CAD build for the part. Positions are in the model's coordinates, mm. A direction names the side the tool comes from. Give positions to 0.01 mm unless a question says otherwise; leave off trailing zeros. Loops run counter-clockwise (first coordinate to the right, second up) from the corner with the lowest first, then second, coordinate; pieces in that order, holes last. Notation, with made-up numbers: (27, 7.25) - (33, 7.25) arc R13 ccw to (33, 19.25) - close; hole circle Ø2 at (36, 40.25). An arc over 180 degrees is marked (long way). Return JSON: item names as keys, results as strings.
from build123d import *

# Parameters (mm, degrees)
SKETCH1_R                = 143
SKETCH1_R_2              = 1.25
BOSS_EXTRUDE1_DEPTH      = 3
SKETCH2_R                = 1.85
BOSS_EXTRUDE2_DEPTH      = 3
FILLET1_R                = 30
CIRPATTERN1_COUNT        = 6
FILLET1_OF_CIRPATTERN1_R = 30
BOSS_EXTRUDE4_DEPTH      = 3
FILLET2_R                = 40


with BuildPart() as part:
    # Sketch1 → Boss-Extrude1 (new body)
    with BuildSketch(Plane.XY):
        Circle(SKETCH1_R)
        Circle(SKETCH1_R_2, mode=Mode.SUBTRACT)
    extrude(amount=BOSS_EXTRUDE1_DEPTH)

    # Sketch2 → Boss-Extrude2 (add)
    with BuildSketch(Plane.XY.offset(3)):
        with BuildLine():
            Line((-136, -8), (-150, -8))
            ThreePointArc((-150, -8), (-158, 0), (-150, 8))
            Line((-150, 8), (-136, 8))
            ThreePointArc((-136, 8), (-128, 0), (-136, -8))
        make_face()
        with Locations((-150, 0)):
            Circle(SKETCH2_R, mode=Mode.SUBTRACT)
    boss_extrude2 = extrude(amount=-BOSS_EXTRUDE2_DEPTH)

    # Fillet1
    fillet1_edges = [part.edges().sort_by_distance(p)[0] for p in [
        (-142.776048411, 8, 1.5),
        (-142.776048411, -8, 1.5),
    ]]
    fillet(fillet1_edges, radius=FILLET1_R)

    # CirPattern1: Boss-Extrude2 ×6 about axis
    cirpattern1_axis = Axis((0, 0, 0), (0, 0, 1))
    for i in range(1, CIRPATTERN1_COUNT):
        add(boss_extrude2.rotate(cirpattern1_axis, i * 360 / CIRPATTERN1_COUNT))

    # Fillet1 of CirPattern1
    fillet1_of_cirpattern1_edges = [part.edges().sort_by_distance(p)[0] for p in [
        (-78.316227436, -119.647684976, 1.5),
        (-64.459820975, -127.647684976, 1.5),
        (64.459820975, -127.647684976, 1.5),
        (78.316227436, -119.647684976, 1.5),
        (142.776048411, -8, 1.5),
        (142.776048411, 8, 1.5),
        (78.316227436, 119.647684976, 1.5),
        (64.459820975, 127.647684976, 1.5),
        (-64.459820975, 127.647684976, 1.5),
        (-78.316227436, 119.647684976, 1.5),
    ]]
    fillet(fillet1_of_cirpattern1_edges, radius=FILLET1_OF_CIRPATTERN1_R)

    # Sketch6 → Boss-Extrude4 (add)
    with BuildSketch(Plane.XY.offset(3)):
        with BuildLine():
            Line((-25, 150), (25, 150))
            ThreePointArc((25, 150), (32, 143), (25, 136))
            Line((25, 136), (-25, 136))
            ThreePointArc((-25, 136), (-32, 143), (-25, 150))
        make_face()
    extrude(amount=-BOSS_EXTRUDE4_DEPTH)

    # Fillet2
    # the kernel refuses this fillet: 40 mm, written as the material it adds along each edge
    with BuildSketch(Plane(origin=(31.105412767, 139.575976789, 3), x_dir=(0.9617682057549536, -0.27386478123135344, 0), z_dir=(0, 0, -1))) as fillet2_piece_1:
        with BuildLine():
            CenterArc((20.599589027, -39.801292998), FILLET2_R, 95.71339394, 29.960885515)
            ThreePointArc((-2.727475038, -7.307476939), (-0.251629619, -4.068826545), (0, 0))
            ThreePointArc((0, 0), (8.308747323, -0.241586175), (16.617494645, 0))
        make_face()
    extrude(amount=3)
    with BuildSketch(Plane(origin=(-31.105412767, 139.575976789, 3), x_dir=(-0.9617682057549533, -0.27386478123135494, 0), z_dir=(0, 0, -1))) as fillet2_piece_2:
        with BuildLine():
            CenterArc((20.599589027, 39.801292998), FILLET2_R, 234.325720545, 29.960885515)
            ThreePointArc((-2.727475038, 7.307476939), (-0.251629619, 4.068826545), (0, 0))
            ThreePointArc((0, 0), (8.308747323, 0.241586175), (16.617494645, 0))
        make_face()
    extrude(amount=3)


solid = part.part
1. Cut at B-B, the plane x = 111. Write the cut outline in (y, z).
Values follow:
{"outline": "(-90.16, 0) - (90.16, 0) - (90.16, 3) - (-90.16, 3) - close"}
2. Cut at A-A, the plane z = 1.2. Give the number of separate pieces and of enclosed holes in the cut face, plus the area to 3 significant figures.
Values follow:
{"separate pieces": "1", "enclosed holes": "7", "area": "66,700 mm²"}
3. Which spindle directions (+Z, -Z, +X, -X, +Y, -Y) get a long thin tool onto all of the face, cutting with end or side? Do faces 4 (the face through (38.09, 140.01, 1.52)), 5 (the face through (-123.504, 72.081, 1.479)). Say none if no direction does.
Values follow:
{"face 4": "+Z, -Z, +Y", "face 5": "+Z, -Z, -X, +Y"}
4. Pull direction X, two halves, no side cores. Call faces 1 (the face through (124.176, 70.917, 1.479)), 2 (the face through (78.9, 136.89, 1.52)), 3 (the face through (-3, 1, 3)): +X half, -X half, draft (parallel to the pull), parting line (faces both ways), or undercut.
Values follow:
{"face 1": "+X half", "face 2": "undercut", "face 3": "draft"}
5. Drill centre lines: probe 1 along Y at (x, z) = (-75, 2.1); probe 2 along Y at (x, z) = (0, 2.1); probe 3 along X at (y, z) = (0.5, 0.8). Where is each one in solid material? Low to high.
Values follow:
{"probe 1": "y = -137.9 to -131.75, -128.05 to 128.05, 131.75 to 137.9", "probe 2": "y = -143 to -1.25, 1.25 to 150", "probe 3": "x = -157.98 to -151.78, -148.22 to -1.15, 1.15 to 148.22, 151.78 to 157.98"}
6. Cut at C-C, the plane y = 84. Write the cut outline in (x, z).
Values follow:
{"outline": "(-115.73, 0) - (115.73, 0) - (115.73, 3) - (-115.73, 3) - close"}
7. Drop flat-ended pins along their axis: P1, Ø5, axis at x = 75, y = 129.9, coming from the -Z side; P2, Ø1.5, axis at x = 68, z = 0.5, coming from the -Y side; P3, Ø1.5, axis at y = -91, z = 2.5, coming from the +X side. Give the stop position or say it passes through.
Values follow:
{"P1": "stops at z = 0", "P2": "stops at y = -135.76", "P3": "stops at x = 110.92"}
